Autodesk Inventor part; units mm, degrees
ref_plane "YZ Plane" through (0, 0, 0) normal (1, 0, 0) x (0, 1, 0)
ref_plane "XZ Plane" through (0, 0, 0) normal (0, 1, 0) x (-1, 0, 0)
ref_plane "XY Plane" through (0, 0, 0) normal (0, 0, 1) x (1, 0, 0)
sketch "Skizze1" plane through (0, 0, 0) normal (0, 1, 0) x (-1, 0, 0)
  line L0 (8.2, -1.8) -> (8.2, -14.2)
  line L1 (8.2, -14.2) -> (-0.2, -14.2)
  line L2 (-0.2, -14.2) -> (-0.2, -1.8)
  line L3 (-7, 5) -> (15, 5)
  line L4 (15, 5) -> (15, -21)
  line L5 (15, -21) -> (-7, -21)
  line L6 (-7, -21) -> (-7, 5)
  line L7 (8.2, -1.8) -> (-0.2, -1.8)
  line L8 (13.2, 3.2) -> (-5.2, 3.2)
  line L9 (-5.2, 3.2) -> (-5.2, -19.2)
  line L10 (-5.2, -19.2) -> (13.2, -19.2)
  line L11 (13.2, -19.2) -> (13.2, 3.2)
  point P0 (0, 0)
  point P1 (8, 0)
  point P2 (4, 0)
  point P3 (4, 5)
  point P4 (4, -14.2)
  point P5 (13.2, -8)
  point P6 (8.2, -8)
  point P7 (4, -19.2)
  point P8 (-5.2, -8)
  dimension "d2" = 6.8
  dimension "d3" = 6.8
  dimension "d56" = 26
  dimension "d57" = 22
  dimension "d58" = 6.8
  dimension "d59" = 6.8
  dimension "d61" = 5
  dimension "d62" = 5
  dimension "d63" = 5
  dimension "d65" = 1.8
  dimension "d66" = 0.2
  dimension "d67" = 5
extrude "Extrusion1" add sketch "Skizze1" along normal blind 10 contours L11 L10 L9 L8
sketch "Skizze2" plane through (0, 0, 0) normal (0, -1, 0) x (1, 0, 0)
  line L0 (23, 19) -> (-31, 19)
  line L1 (-31, 19) -> (-31, -35)
  line L2 (-31, -35) -> (23, -35)
  line L3 (23, -35) -> (23, 19)
  line L4 (-15, -21) -> (-15, 5)
  line L5 (7, -21) -> (-15, -21)
  line L6 (7, 5) -> (7, -21)
  line L7 (-15, 5) -> (7, 5)
  point P0 (0, 0)
  dimension "d11" = 16
  dimension "d12" = 14
  dimension "d13" = 16
  dimension "d14" = 14
  dimension "d35" = 54
  dimension "d36" = 54
extrude "Extrusion2" add sketch "Skizze2" along normal blind 5 contours L3 L2 L1 L0 | L4 L7 L6 L5
sketch "Skizze4" plane through (0, 0, 0) normal (0, 1, 0) x (1, 0, 0)
  line L0 (23, 35) -> (23, -19)
  line L1 (-31, 35) -> (23, 35)
  line L2 (23, -19) -> (-31, -19)
  line L3 (-31, -19) -> (-31, 35)
  point P0 (0, 0)
  point P1 (16, 28)
  point P2 (16, -12)
  point P3 (-24, -12)
  point P4 (-24, 28)
  dimension "d44" = 7
  dimension "d45" = 7
  dimension "d46" = 7
  dimension "d47" = 7
  dimension "d48" = 7
  dimension "d49" = 7
  dimension "d50" = 7
  dimension "d51" = 7
  dimension "d52" = 40
  dimension "d53" = 40
  dimension "d54" = 40
  dimension "d55" = 40
hole "Bohrung1" at (16, 0, -28) at (16, 0, 12) at (-24, 0, 12) at (-24, 0, -28) direction (0, -1, 0) diameter 8.5 depth 5
chamfer "Fasen5" distance 10 angle 21.8 1 edges at (-8.2, 10, -8) measured on face at (-8.2, 3.3333, -5.9333)
chamfer "Fasen6" distance 10 angle 21.8 1 edges at (-4, 10, -1.8) measured on face at (-2.6, 3.3335, -1.8)
chamfer "Fasen7" distance 10 angle 21.8 1 edges at (0.2, 10, -8) measured on face at (0.2, 3.3335, -10.0667)
chamfer "Fasen8" distance 10 angle 21.8 1 edges at (-4, 10, -14.2) measured on face at (-2.6, 6.6668, -14.2)
properties part number "Magazin_1_3D-Druck"
Build history of the part. All positions in model axes, mm. A direction names the side the tool comes from. Coordinates: 2 decimals unless noted, no trailing zeros. Write each loop counter-clockwise with the first axis right and the second up, starting at its lowest first coordinate (ties: lowest second). Pieces come first, ordered by that corner, then holes.
1. 3-axis set-ups, long thin cutter, end or side, ignore diameter. For faces 1 (the flat face through (-31, -2, -8)), 2 (the flat face through (-4, 5, -19.2)), 3 (the flat face through (-13.2, 5, -8)), 4 (the flat face through (2.228, 5.07, -7.857)): which of +Z, -Z, +X, -X, +Y, -Y reach the whole face in a straight line?
Answer block:
face 1: +Z, -Z, -X, +Y, -Y
face 2: -Z, +X, -X, +Y
face 3: +Z, -Z, -X, +Y
face 4: +Y
2. Band-saw the part on B-B, the plane x = -24. Give the cut face in (y, z).
Answer block:
outline: (-5, -35) - (0, -35) - (0, -32.25) - (-5, -32.25) - close; (-5, -23.75) - (0, -23.75) - (0, 7.75) - (-5, 7.75) - close; (-5, 16.25) - (0, 16.25) - (0, 19) - (-5, 19) - close
3. Band-saw the part on A-A, the plane z = -30. Give the cut face in (x, y), and give its area (3 significant figures).
Answer block:
outline: (-31, -5) - (-27.75, -5) - (-27.75, 0) - (-31, 0) - close; (-20.25, -5) - (12.25, -5) - (12.25, 0) - (-20.25, 0) - close; (19.75, -5) - (23, -5) - (23, 0) - (19.75, 0) - close
area: 195 mm2
4. Drop flat-ended pins along their axis: pin 1 (11 mm diameter, centred on x = -24, z = 12, fed in from +Y); pin 2 (1 mm diameter, centred on x = 2.5, y = 2.5, fed in from -Z); pin 3 (8 mm diameter, centred on y = 6.5, z = -12, fed in from -X). Give the stop position or say it passes through.
Answer block:
pin 1: stops at y = 0
pin 2: stops at z = -19.2
pin 3: stops at x = -13.2
5. Band-saw the part on C-C, the plane y = -2. Give the cut face in (x, z), and give its area (3 significant figures).
Answer block:
outline: (-31, -35) - (23, -35) - (23, 19) - (-31, 19) - close; hole circle Ø8.5 at (-24, -28); hole circle Ø8.5 at (-24, 12); hole circle Ø8.5 at (16, -28); hole circle Ø8.5 at (16, 12)
area: 2,690 mm2
6. Pull direction Z, two halves, no side cores. Call faces 5 (the flat face through (-4, 5, 3.2)), 6 (the cylindrical face through (18.59, -2.54, -31.37)), 7 (the flat face through (23, -2, -8)): released by +Z, released by -Z, zero draft, split by the parting line, or undercut.
Answer block:
face 5: released by +Z
face 6: undercut
face 7: zero draft
7. Drill centre lines: probe 1 along Z at (x, y) = (16, -2.4); probe 2 along X at (y, z) = (-1.6, -28); probe 3 along X at (y, z) = (-2, 10.5). Where is each one in solid material? Low to high.
Answer block:
probe 1: z = -35 to -32.25, -23.75 to 7.75, 16.25 to 19
probe 2: x = -31 to -28.25, -19.75 to 11.75, 20.25 to 23
probe 3: x = -31 to -27.98, -20.02 to 12.02, 19.98 to 23
